Here's how the part is built. I have some questions about the finished solid (model axes, mm). Give positions to 0.01 mm unless a question says otherwise; leave off trailing zeros. Write each loop counter-clockwise with the first axis right and the second up, starting at its lowest first coordinate (ties: lowest second). Pieces come first, ordered by that corner, then holes. Notation, with made-up numbers: (-15.5, 34) - (1.5, 34) arc R27 cw to (1.5, 59) - close; hole circle Ø9 at (69.25, 16.25). An arc over 180 degrees is marked (long way). One line per item, written item: value. Start each with the question number.
1) Please list where this line runs through material, in increasing order: L1, parallel to Y at x = -88, z = -0.25. Write a range as [from, to].
2) Imagine slicing it at C-C on z = -1.6. Write out the boundary of the cut face in (x, y).
3) Imagine slicing it at A-A on y = 60. Write out the boundary of the cut face in (x, z).
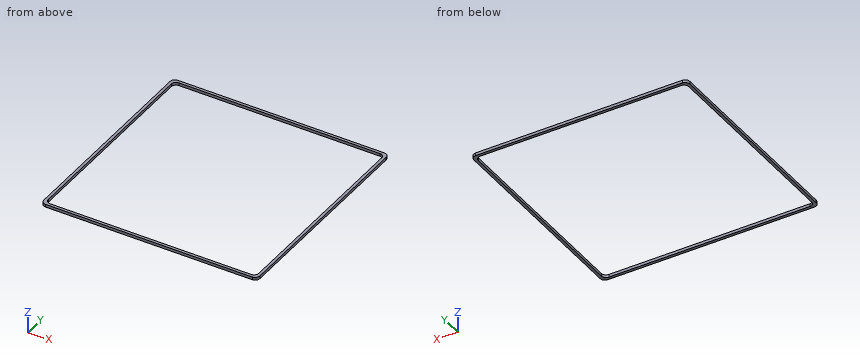
Autodesk Inventor part; units mm, degrees
ref_plane "YZ Plane" through (0, 0, 0) normal (1, 0, 0) x (0, 1, 0)
ref_plane "XZ Plane" through (0, 0, 0) normal (0, 1, 0) x (-1, 0, 0)
ref_plane "XY Plane" through (0, 0, 0) normal (0, 0, 1) x (1, 0, 0)
sketch "Sketch1" plane through (0, 0, 0) normal (0, 0, 1) x (1, 0, 0)
  line L0 (-115, 115) -> (115, 115)
  line L1 (115, 115) -> (115, -115)
  line L2 (115, -115) -> (-115, -115)
  line L3 (-115, -115) -> (-115, 115)
  line L4 (112, 112) -> (-112, 112)
  line L5 (-112, 112) -> (-112, -112)
  line L6 (-112, -112) -> (112, -112)
  line L7 (112, -112) -> (112, 112)
  point P0 (0, 0)
  dimension "d0" = 230
  dimension "d1" = 230
  dimension "d2" = 115
  dimension "d3" = 115
  dimension "d4" = 3
extrude "Extrusion1" add sketch "Sketch1" against normal blind 3
fillet "Fillet1" radius 5 8 edges at (-115, 115, -1.5) (-112, 112, -1.5) (-112, -112, -1.5) (-115, -115, -1.5) (115, -115, -1.5) (112, -112, -1.5) (115, 115, -1.5) (112, 112, -1.5)
equation "\"d1\" = d0"
properties part number "border"
Numbers:
1. L1: [-115, -112], [112, 115]
2. outline: (-115, -110) arc R5 ccw to (-110, -115) - (110, -115) arc R5 ccw to (115, -110) - (115, 110) arc R5 ccw to (110, 115) - (-110, 115) arc R5 ccw to (-115, 110) - close; hole (-112, -107) arc R5 ccw to (-107, -112) - (107, -112) arc R5 ccw to (112, -107) - (112, 107) arc R5 ccw to (107, 112) - (-107, 112) arc R5 ccw to (-112, 107) - close
3. outline: (-115, -3) - (-112, -3) - (-112, 0) - (-115, 0) - close; (112, -3) - (115, -3) - (115, 0) - (112, 0) - close
